```python
from build123d import *

# Parameters (mm, degrees)
SKETCH1_W           = 155
SKETCH1_H           = 40
BOSS_EXTRUDE1_DEPTH = 15
SKETCH2_R           = 11
CUT_EXTRUDE1_DEPTH  = 7
CUT_EXTRUDE2_START  = -15
SKETCH3_R           = 6.070786999
CUT_EXTRUDE2_DEPTH  = 8


with BuildPart() as part:
    # Sketch1 → Boss-Extrude1 (new body)
    with BuildSketch(Plane.XY):
        Rectangle(SKETCH1_W, SKETCH1_H)
    extrude(amount=BOSS_EXTRUDE1_DEPTH)

    # Sketch2 → Cut-Extrude1 (cut)
    with BuildSketch(Plane(origin=(0, 0, 0), x_dir=(-1, 0, 0), z_dir=(0, 0, -1))):
        Circle(SKETCH2_R)
    extrude(amount=-CUT_EXTRUDE1_DEPTH, mode=Mode.SUBTRACT)

    # Sketch3 → Cut-Extrude2 (cut)
    with BuildSketch(Plane(origin=(0, 0, 0), x_dir=(-1, 0, 0), z_dir=(0, 0, -1)).offset(CUT_EXTRUDE2_START)):
        Circle(SKETCH3_R)
    extrude(amount=CUT_EXTRUDE2_DEPTH, mode=Mode.SUBTRACT)


solid = part.part
```
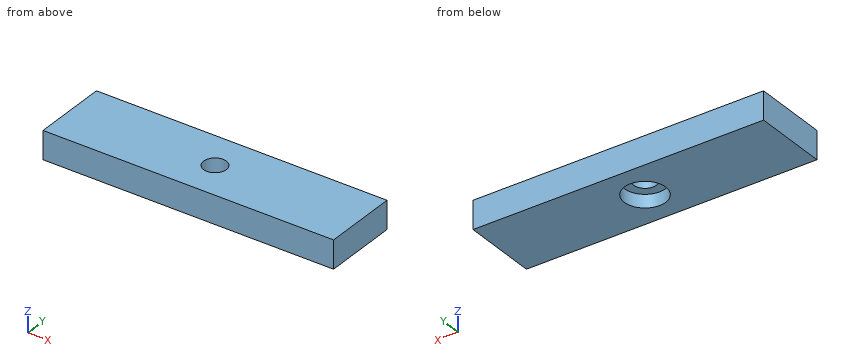
Source: CAD feature listing. Evaluate the final solid. Frame: model axes, mm. Coordinates: 2 decimals unless noted, no trailing zeros. Write each loop counter-clockwise with the first axis right and the second up, starting at its lowest first coordinate (ties: lowest second). Pieces come first, ordered by that corner, then holes. Notation, with made-up numbers: (28.25, -7) -> (48.25, -7) arc R28 cw to (48.25, 21) -> close; hole circle Ø4 at (2.25, 69.5). An arc over 180 degrees is marked (long way). Return JSON: item names as keys, results as strings. Group by question number.
1) Section query A-A, the plane x = 0. Return loops of the section in (y, z), plus the area to 3 significant figures.
2) Section query D-D, the plane z = 13.5. Return loops of the section in (x, y), plus the area to 3 significant figures.
3) Contact query for a flat-ended pin moving along its axis: P1, Ø11, axis at x = -0.5, y = 4, coming from the -Z side. Output: stop coordinate, or through.
4) Ray query, line 1 along Y through (x, z) = (0, 4.75); line 2 along X through (y, z) = (0.5, 12.75); line 3 along Y through (x, z) = (0, 11.5). Return the intervals inside material, ascending.
5) Section query C-C, the plane y = 0. Return loops of the section in (x, z), plus the area to 3 significant figures.
6) Section query B-B, the plane z = 4. Return loops of the section in (x, y), plus the area to 3 significant figures.
From the geometry:
{
 "1": {"outline": "(-20, 0) -> (-11, 0) -> (-11, 7) -> (-6.07, 7) -> (-6.07, 15) -> (-20, 15) -> close; (6.07, 7) -> (11, 7) -> (11, 0) -> (20, 0) -> (20, 15) -> (6.07, 15) -> close", "area": "349 mm²"},
 "2": {"outline": "(-77.5, -20) -> (77.5, -20) -> (77.5, 20) -> (-77.5, 20) -> close; hole circle Ø12.14 at (0, 0)", "area": "6,080 mm²"},
 "3": {"P1": "z = 7"},
 "4": {"line 1": "-20 to -11, 11 to 20", "line 2": "-77.5 to -6.05, 6.05 to 77.5", "line 3": "-20 to -6.07, 6.07 to 20"},
 "5": {"outline": "(-77.5, 0) -> (-11, 0) -> (-11, 7) -> (-6.07, 7) -> (-6.07, 15) -> (-77.5, 15) -> close; (6.07, 7) -> (11, 7) -> (11, 0) -> (77.5, 0) -> (77.5, 15) -> (6.07, 15) -> close", "area": "2,070 mm²"},
 "6": {"outline": "(-77.5, -20) -> (77.5, -20) -> (77.5, 20) -> (-77.5, 20) -> close; hole circle Ø22 at (0, 0)", "area": "5,820 mm²"}
}
